```python
from build123d import *

# Parameters (mm, degrees)
SKETCH1_R               = 27.5
BOSS_EXTRUDE1_DEPTH     = 16
BOSS_EXTRUDE2_START     = -4
SKETCH1_3_R             = 27.5
BOSS_EXTRUDE2_DEPTH     = 4
CUT_EXTRUDE1_DEPTH      = 43.053537307
CUT_EXTRUDE1_DEPTH_BACK = 43.053537307
SKETCH1_5_R             = 11.2
SKETCH6_R               = 3
SKETCH6_R_2             = 1.6
BOSS_EXTRUDE6_DEPTH     = 6
BOSS_EXTRUDE6_2_DEPTH   = 6
BOSS_EXTRUDE6_3_DEPTH   = 6
BOSS_EXTRUDE6_4_DEPTH   = 6
BOSS_EXTRUDE8_START     = -6
SKETCH8_R               = 1.6
BOSS_EXTRUDE8_DEPTH     = 6


with BuildPart() as part:
    # Sketch1 → Boss-Extrude1 (new body)
    with BuildSketch(Plane(origin=(0, 0, 0), x_dir=(1, 0, 0), z_dir=(0, 1, 0))):
        with Locations(Location((0, 0, 0), (0, 0, 270))):
            Circle(SKETCH1_R)
        with BuildLine():
            ThreePointArc((1.140791464, 24.973958333), (7.043313921, 23.98732434), (12.542246399, 21.626189106))
            ThreePointArc((12.542246399, 21.626189106), (12.164418393, 18.928204489), (14.461636098, 20.392672247))
            ThreePointArc((14.461636098, 20.392672247), (18.893739359, 16.371518349), (22.24320965, 11.412257642))
            ThreePointArc((22.24320965, 11.412257642), (20.466719895, 9.346837793), (23.191013452, 9.33685681))
            ThreePointArc((23.191013452, 9.33685681), (24.745536047, 3.557870957), (24.882111, -2.424984989))
            ThreePointArc((24.882111, -2.424984989), (22.270982442, -3.202083861), (24.557407894, -4.683344693))
            ThreePointArc((24.557407894, -4.683344693), (22.740799884, -10.385375325), (19.621117916, -15.49231202))
            ThreePointArc((19.621117916, -15.49231202), (17.004365423, -14.734366514), (18.126998845, -17.216617347))
            ThreePointArc((18.126998845, -17.216617347), (13.516020436, -21.031338321), (8.13055853, -23.640939448))
            ThreePointArc((8.13055853, -23.640939448), (6.338982529, -21.588591906), (5.941395741, -24.28373564))
            ThreePointArc((5.941395741, -24.28373564), (0, -25), (-5.941395741, -24.28373564))
            ThreePointArc((-5.941395741, -24.28373564), (-6.338982529, -21.588591906), (-8.13055853, -23.640939448))
            ThreePointArc((-8.13055853, -23.640939448), (-13.516020436, -21.031338321), (-18.126998845, -17.216617347))
            ThreePointArc((-18.126998845, -17.216617347), (-17.004365423, -14.734366514), (-19.621117916, -15.49231202))
            ThreePointArc((-19.621117916, -15.49231202), (-22.740799884, -10.385375325), (-24.557407894, -4.683344693))
            ThreePointArc((-24.557407894, -4.683344693), (-22.270982442, -3.202083861), (-24.882111, -2.424984989))
            ThreePointArc((-24.882111, -2.424984989), (-24.745536047, 3.557870957), (-23.191013452, 9.33685681))
            ThreePointArc((-23.191013452, 9.33685681), (-20.466719895, 9.346837793), (-22.24320965, 11.412257642))
            ThreePointArc((-22.24320965, 11.412257642), (-18.893739359, 16.371518349), (-14.461636098, 20.392672247))
            ThreePointArc((-14.461636098, 20.392672247), (-12.164418393, 18.928204489), (-12.542246399, 21.626189106))
            ThreePointArc((-12.542246399, 21.626189106), (-7.043313921, 23.98732434), (-1.140791464, 24.973958333))
            ThreePointArc((-1.140791464, 24.973958333), (0, 22.5), (1.140791464, 24.973958333))
        make_face(mode=Mode.SUBTRACT)
    extrude(amount=BOSS_EXTRUDE1_DEPTH)

    # Sketch1<3> → Boss-Extrude2 (add)
    with BuildSketch(Plane(origin=(0, 0, 0), x_dir=(1, 0, 0), z_dir=(0, 1, 0)).offset(BOSS_EXTRUDE2_START)):
        with Locations(Location((0, 0, 0), (0, 0, 270))):
            Circle(SKETCH1_3_R)
    extrude(amount=BOSS_EXTRUDE2_DEPTH)

    # Sketch1<5> → Cut-Extrude1 (cut, two sides: drawn at the far end of the back side and taken through both)
    with BuildSketch(Plane(origin=(0, 0, 0), x_dir=(1, 0, 0), z_dir=(0, 1, 0)).offset(-CUT_EXTRUDE1_DEPTH_BACK)):
        with Locations(Location((0, 0, 0), (0, 0, 270))):
            Circle(SKETCH1_5_R)
    extrude(amount=CUT_EXTRUDE1_DEPTH + CUT_EXTRUDE1_DEPTH_BACK, mode=Mode.SUBTRACT)



with BuildPart() as body_2:
    # Sketch6 → Boss-Extrude6 (new body)
    with BuildSketch(Plane(origin=(0, 10, 0), x_dir=(1, 0, 0), z_dir=(0, 1, 0))):
        with Locations(Location((-30.5, 0, 0), (0, 0, 270))):
            Circle(SKETCH6_R)
        with Locations(Location((-30.5, 0, 0), (0, 0, 270))):
            Circle(SKETCH6_R_2, mode=Mode.SUBTRACT)
    extrude(amount=BOSS_EXTRUDE6_DEPTH)


with BuildPart() as body_3:
    # Sketch6 → Boss-Extrude6 2 (new body)
    with BuildSketch(Plane(origin=(0, 10, 0), x_dir=(1, 0, 0), z_dir=(0, 1, 0))):
        with Locations(Location((0, 30.5, 0), (0, 0, 270))):
            Circle(SKETCH6_R)
        with Locations(Location((0, 30.5, 0), (0, 0, 270))):
            Circle(SKETCH6_R_2, mode=Mode.SUBTRACT)
    extrude(amount=BOSS_EXTRUDE6_2_DEPTH)


with BuildPart() as body_4:
    # Sketch6 → Boss-Extrude6 3 (new body)
    with BuildSketch(Plane(origin=(0, 10, 0), x_dir=(1, 0, 0), z_dir=(0, 1, 0))):
        with Locations(Location((30.5, 0, 0), (0, 0, 270))):
            Circle(SKETCH6_R)
        with Locations(Location((30.5, 0, 0), (0, 0, 270))):
            Circle(SKETCH6_R_2, mode=Mode.SUBTRACT)
    extrude(amount=BOSS_EXTRUDE6_3_DEPTH)


with BuildPart() as body_5:
    # Sketch6 → Boss-Extrude6 4 (new body)
    with BuildSketch(Plane(origin=(0, 10, 0), x_dir=(1, 0, 0), z_dir=(0, 1, 0))):
        with Locations(Location((0, -30.5, 0), (0, 0, 270))):
            Circle(SKETCH6_R)
        with Locations(Location((0, -30.5, 0), (0, 0, 270))):
            Circle(SKETCH6_R_2, mode=Mode.SUBTRACT)
    extrude(amount=BOSS_EXTRUDE6_4_DEPTH)


with BuildPart() as part_1:
    add(part.part)

    add(body_2.part)  # Boss-Extrude8 merges body 2

    add(body_3.part)  # Boss-Extrude8 merges body 3

    add(body_4.part)  # Boss-Extrude8 merges body 4

    add(body_5.part)  # Boss-Extrude8 merges body 5
    # Sketch8 → Boss-Extrude8 (add)
    # profile 1 of 4: a face of its own
    with BuildSketch(Plane(origin=(0, 16, 0), x_dir=(1, 0, 0), z_dir=(0, 1, 0)).offset(BOSS_EXTRUDE8_START)):
        with BuildLine():
            ThreePointArc((-32.31166617, -2.391205906), (-28.079459744, -6.502708785), (-24.971529598, -11.518364013))
            ThreePointArc((-24.971529598, -11.518364013), (-27.5, 0), (-24.971529598, 11.518364013))
            ThreePointArc((-24.971529598, 11.518364013), (-28.079459744, 6.502708785), (-32.31166617, 2.391205906))
            ThreePointArc((-32.31166617, 2.391205906), (-33.5, 0), (-32.31166617, -2.391205906))
        make_face()
        with Locations(Location((-30.5, 0, 0), (0, 0, 270))):
            Circle(SKETCH8_R, mode=Mode.SUBTRACT)
    # profile 2 of 4: a face of its own
    with BuildSketch(Plane(origin=(0, 16, 0), x_dir=(1, 0, 0), z_dir=(0, 1, 0)).offset(BOSS_EXTRUDE8_START)):
        with BuildLine():
            ThreePointArc((-2.391205906, 32.31166617), (-6.502708785, 28.079459744), (-11.518364013, 24.971529598))
            ThreePointArc((-11.518364013, 24.971529598), (0, 27.5), (11.518364013, 24.971529598))
            ThreePointArc((11.518364013, 24.971529598), (6.502708785, 28.079459744), (2.391205906, 32.31166617))
            ThreePointArc((2.391205906, 32.31166617), (0, 33.5), (-2.391205906, 32.31166617))
        make_face()
        with Locations(Location((0, 30.5, 0), (0, 0, 270))):
            Circle(SKETCH8_R, mode=Mode.SUBTRACT)
    # profile 3 of 4: a face of its own
    with BuildSketch(Plane(origin=(0, 16, 0), x_dir=(1, 0, 0), z_dir=(0, 1, 0)).offset(BOSS_EXTRUDE8_START)):
        with BuildLine():
            ThreePointArc((32.31166617, 2.391205906), (28.079459744, 6.502708785), (24.971529598, 11.518364013))
            ThreePointArc((24.971529598, 11.518364013), (27.5, 0), (24.971529598, -11.518364013))
            ThreePointArc((24.971529598, -11.518364013), (28.079459744, -6.502708785), (32.31166617, -2.391205906))
            ThreePointArc((32.31166617, -2.391205906), (33.5, 0), (32.31166617, 2.391205906))
        make_face()
        with Locations(Location((30.5, 0, 0), (0, 0, 270))):
            Circle(SKETCH8_R, mode=Mode.SUBTRACT)
    # profile 4 of 4: a face of its own
    with BuildSketch(Plane(origin=(0, 16, 0), x_dir=(1, 0, 0), z_dir=(0, 1, 0)).offset(BOSS_EXTRUDE8_START)):
        with BuildLine():
            ThreePointArc((2.391205906, -32.31166617), (6.502708785, -28.079459744), (11.518364013, -24.971529598))
            ThreePointArc((11.518364013, -24.971529598), (0, -27.5), (-11.518364013, -24.971529598))
            ThreePointArc((-11.518364013, -24.971529598), (-6.502708785, -28.079459744), (-2.391205906, -32.31166617))
            ThreePointArc((-2.391205906, -32.31166617), (0, -33.5), (2.391205906, -32.31166617))
        make_face()
        with Locations(Location((0, -30.5, 0), (0, 0, 270))):
            Circle(SKETCH8_R, mode=Mode.SUBTRACT)
    extrude(amount=BOSS_EXTRUDE8_DEPTH)


solid = part_1.part
```
For this review, take the finished solid that the model builds, in its own axes (mm). A direction names the side the tool comes from. Round coordinates to 2 decimals unless told otherwise and drop trailing zeros. Loops run counter-clockwise (first coordinate to the right, second up) from the corner with the lowest first, then second, coordinate; pieces in that order, holes last.
(1) We need section D-D (z = -15). Give the boundary of the cut face in (x, y).
Returned:
outline: (-23.05, -4) - (23.05, -4) - (23.05, 16) - (20, 16) - (20, 0) - (-20, 0) - (-20, 16) - (-23.05, 16) - close
(2) We need section A-A (x = 30.5). Give the boundary of the cut face in (y, z), plus the area to 3 significant figures.
Returned:
outline: (10, -3.91) - (16, -3.91) - (16, -1.6) - (10, -1.6) - close; (10, 1.6) - (16, 1.6) - (16, 3.91) - (10, 3.91) - close
area: 27.7 mm2
(3) We need section C-C (z = 30.5). Give the boundary of the cut face in (x, y).
Returned:
outline: (-3.91, 10) - (-1.6, 10) - (-1.6, 16) - (-3.91, 16) - close; (1.6, 10) - (3.91, 10) - (3.91, 16) - (1.6, 16) - close
(4) We need section B-B (y = 5.5). Give the boundary of the cut face in (x, z), plus the area to 3 significant figures.
Returned:
outline: circle Ø55 at (0, 0); hole (-24.88, 2.42) arc R25 ccw to (-23.19, -9.34) arc R1.5 cw (long way) to (-22.24, -11.41) arc R25 ccw to (-14.46, -20.39) arc R1.5 cw (long way) to (-12.54, -21.63) arc R25 ccw to (-1.14, -24.97) arc R1.5 cw (long way) to (1.14, -24.97) arc R25 ccw to (12.54, -21.63) arc R1.5 cw (long way) to (14.46, -20.39) arc R25 ccw to (22.24, -11.41) arc R1.5 cw (long way) to (23.19, -9.34) arc R25 ccw to (24.88, 2.42) arc R1.5 cw (long way) to (24.56, 4.68) arc R25 ccw to (19.62, 15.49) arc R1.5 cw (long way) to (18.13, 17.22) arc R25 ccw to (8.13, 23.64) arc R1.5 cw (long way) to (5.94, 24.28) arc R25 ccw to (-5.94, 24.28) arc R1.5 cw (long way) to (-8.13, 23.64) arc R25 ccw to (-18.13, 17.22) arc R1.5 cw (long way) to (-19.62, 15.49) arc R25 ccw to (-24.56, 4.68) arc R1.5 cw (long way) to start
area: 481 mm2
(5) Tool access review of faces 5 (the cylindrical face through (1.209, 3.638, -27.473)), 6 (the flat face through (-18, 16, 15)): name each direction out of +Z, -Z, +X, -X, +Y, -Y from which nothing blocks a thin tool from reaching the whole face with its end or side.
Returned:
face 5: -Y
face 6: +Z, -Z, +X, -X, +Y
(6) Mouldability with a two-part tool opening along Z and no side actions: class faces 1 (the cylindrical face through (-6.44, 12.96, -28.13)), 2 (the cylindrical face through (-28.13, 12.96, 6.44)), 3 (the cylindrical face through (7, 8, -24)), 4 (the cylindrical face through (-24.76, 7.89, -3.47)) as released by +Z, released by -Z, zero draft, split by the parting line, or undercut.
Returned:
face 1: released by -Z
face 2: released by +Z
face 3: undercut
face 4: undercut
(7) Clearance check with flat-ended pins moving along their axes: P1, Ø3.5, axis at x = 0, z = 30.5, coming from the -Y side; P2, Ø4, axis at x = 6, y = 10.5, coming from the +Z side; P3, Ø25, axis at x = 3, z = -5, coming from the +Y side; P4, Ø3, axis at x = 0, z = -30.5, coming from the -Y side. State where each tip first meets the part, or that it passes through.
Returned:
P1: stops at y = 10
P2: stops at z = 30.4
P3: stops at y = 0
P4: passes through
(8) Wall thickness on line 1 along Z through (x, y) = (0, -1.45); line 2 along Y through (x, z) = (5.5, -18): over which ranges is each line inside the solid? List them lowest first.
Returned:
line 1: z = -27.5 to -11.2, 11.2 to 27.5
line 2: y = -4 to 0
